CAD build for the part. Positions are in the model's coordinates, mm. Give positions to 0.01 mm unless a question says otherwise; leave off trailing zeros. Answer as a JSON object with one key per item and string values.
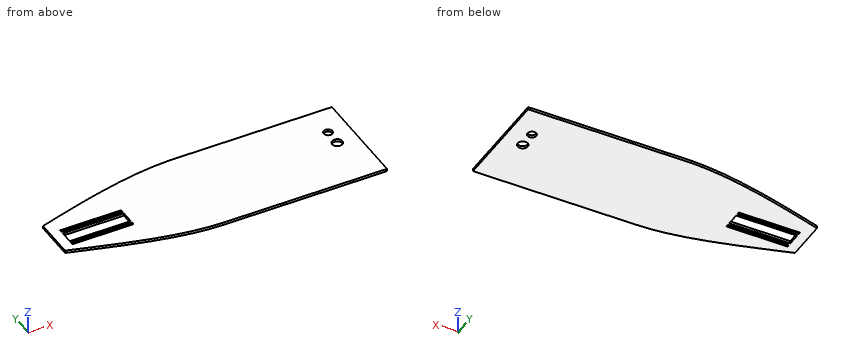
from build123d import *

# Parameters (mm, degrees)
F0_W      = 406.4
F0_H      = 254
F0_R      = 10.795
F1_DEPTH  = 6.35
F2_W      = 101.6
F2_H      = 6.35
F3_DEPTH  = 355.6
F5_DEPTH  = 6.35
F7_DEPTH  = 6.35
F8_W      = 152.4
F8_H      = 31.75
F9_DEPTH  = 6.35
F11_DEPTH = 6.35
F12_W     = 152.4
F12_H     = 6.35
F13_DEPTH = 6.35
F15_DEPTH = 6.35


with BuildPart() as f1:
    # F0 (on Top) → F1 (new body)
    with BuildSketch(Plane.XY):
        with Locations((203.2, 127)):
            Rectangle(F0_W, F0_H)
        with Locations((355.6, 177.8)):
            Circle(F0_R, mode=Mode.SUBTRACT)
    extrude(amount=F1_DEPTH)

    # F2 (on face) → F3 (join)
    with BuildSketch(Plane(origin=(0, 0, 0), x_dir=(0, -1, 0), z_dir=(-1, 0, 0))):
        with Locations((-127, 3.175)):
            Rectangle(F2_W, F2_H)
    extrude(amount=F3_DEPTH)

    # F4 (on face) → F5 (join)
    with BuildSketch(Plane.XY.offset(6.35)):
        with BuildLine():
            Line((0, 177.8), (0, 254))
            add(Edge.make_bspline(
                [(0, 254), (-112.8963902593, 250.5958378315), (-238.5879904032, 212.7161622047), (-355.6, 177.8)],
                knots=[0, 0, 0, 0, 363.6726550072, 363.6726550072, 363.6726550072, 363.6726550072], degree=3))
            Line((-355.6, 177.8), (0, 177.8))
        make_face()
    extrude(amount=-F5_DEPTH)

    # F6 (on face) → F7 (join)
    with BuildSketch(Plane.XY.offset(6.35)):
        with BuildLine():
            add(Edge.make_bspline(
                [(0, 0), (-114.120438695, 0), (-236.8435710669, 41.2505157292), (-355.6, 76.2)],
                knots=[0, 0, 0, 0, 363.6726550072, 363.6726550072, 363.6726550072, 363.6726550072], degree=3))
            Line((0, 0), (0, 76.2))
            Line((0, 76.2), (-355.6, 76.2))
        make_face()
    extrude(amount=-F7_DEPTH)

    # F8 (on face) → F9 (cut)
    with BuildSketch(Plane.XY.offset(6.35)):
        with Locations((-254, 117.475)):
            Rectangle(F8_W, F8_H)
    extrude(amount=-F9_DEPTH, mode=Mode.SUBTRACT)

    # F10 (on face) → F11 (cut)
    with BuildSketch(Plane.XY.offset(6.35)):
        Polygon((-330.2, 146.05), (-330.2, 139.7), (-269.6087956429, 139.7), (-177.8, 139.7), (-177.8, 146.05), align=None)
    extrude(amount=-F11_DEPTH, mode=Mode.SUBTRACT)

    # F12 (on face) → F13 (cut)
    with BuildSketch(Plane.XY.offset(6.35)):
        with Locations((-254, 92.075)):
            Rectangle(F12_W, F12_H)
    extrude(amount=-F13_DEPTH, mode=Mode.SUBTRACT)

    # F14 (on face) → F15 (cut)
    with BuildSketch(Plane.XY.offset(6.35)):
        with BuildLine():
            ThreePointArc((368.3, 135.255), (364.5802561211, 144.2352561211), (355.6, 147.955))
            ThreePointArc((355.6, 147.955), (346.6197438789, 126.2747438789), (368.3, 135.255))
        make_face()
    extrude(amount=-F15_DEPTH, mode=Mode.SUBTRACT)


solid = f1.part
(1) Flat gauge pins, fed straight in: P1, Ø3, axis at x = -251, z = 2.5, coming from the +Y side; P2, Ø3, axis at x = -264.5, z = 4, coming from the -Y side; P3, Ø13, axis at x = 355.6, y = 177.8, coming from the -Z side; P4, Ø2, axis at x = -230, z = 4.5, coming from the -Y side. Where does each tip first touch, or does it go through?
Answer key:
{"P1": "stops at y = 208.74", "P2": "stops at y = 48.68", "P3": "passes through", "P4": "stops at y = 38.95"}
(2) Saw through at A-A, the plane z = 3.25. State how many separate pieces and enclosed holes the cut face has, and give its area (3 significant figures).
Answer key:
{"separate pieces": "1", "enclosed holes": "5", "area": "165,000 mm²"}
(3) Probe L1, parallel to Y at x = 355.6, z = 4.5 (3 decimals); L2, parallel to Y at x = -264.5, z = 6.25; L3, parallel to Y at x = 353.5, z = 2. List the from-to ranges inside material, lowest first. Write a range as [from, to].
Answer key:
{"L1": "y = [0, 122.555], [147.955, 167.005], [188.595, 254]", "L2": "y = [49.11, 88.9], [95.25, 101.6], [133.35, 139.7], [146.05, 204.54]", "L3": "y = [0, 122.73], [147.78, 167.21], [188.39, 254]"}
